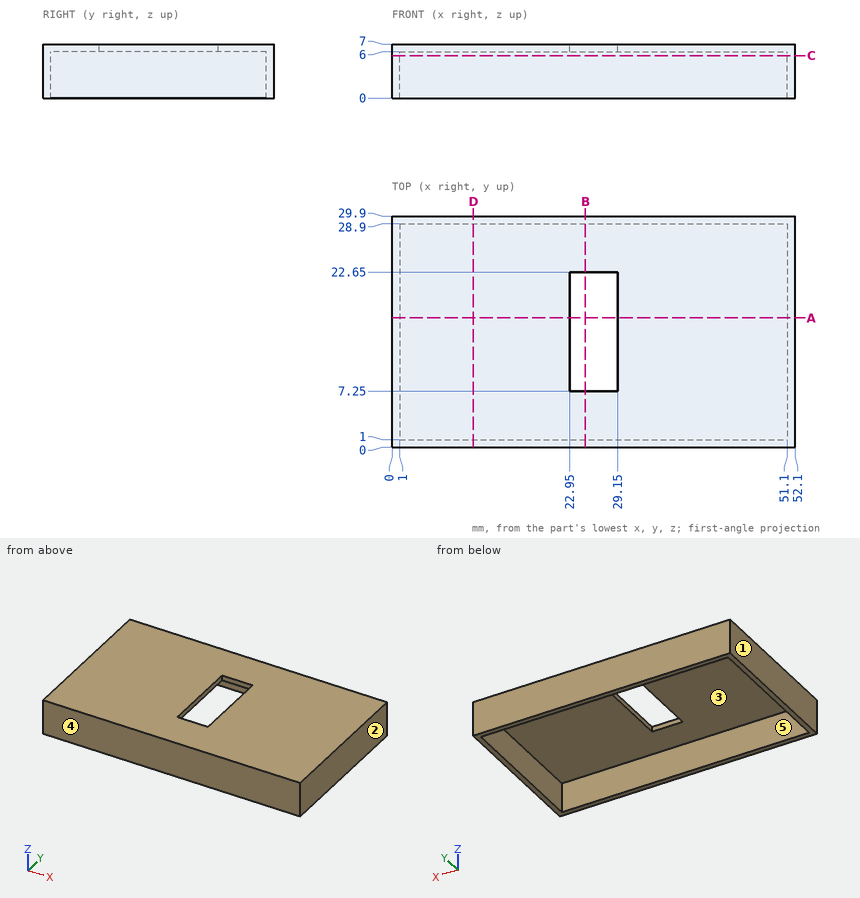
Could you check a few things on this drawing? It's one solid part, dimensions in mm from its lowest x, y, z. A direction names the side the tool comes from. Give positions to 0.01 mm unless a question says otherwise; leave off trailing zeros. Write each loop counter-clockwise with the first axis right and the second up, starting at its lowest first coordinate (ties: lowest second). Pieces come first, ordered by that corner, then holes. Notation, with made-up numbers: (-14.75, 74.25) -> (4.25, 74.25) arc R19 cw to (4.25, 93.25) -> close; hole circle Ø10 at (-18.5, 49). An arc over 180 degrees is marked (long way). Answer as a JSON object with one key per item and string values.
Q1. Will this pin go through, and if not, where does the flat tip stop? pin 1 Ø6 at (x, y) = (44, 7.5) entering from -Z.
Taken from the geometry:
{"pin 1": "stops at z = 6"}
Q2. Suppose I cut it at D-D on x = 10.5. Write out the boundary of the cut face in (y, z), then the cut area to 3 significant figures.
Taken from the geometry:
{"outline": "(0, 0) -> (1, 0) -> (1, 6) -> (28.9, 6) -> (28.9, 0) -> (29.9, 0) -> (29.9, 7) -> (0, 7) -> close", "area": "41.9 mm²"}
Q3. We'd pull the mould along X, two halves only. Please class the marked faces 1, 2 and 3: released by +X, released by -X, zero draft, split by the parting line, or undercut.
Taken from the geometry:
{"face 1": "released by -X", "face 2": "released by +X", "face 3": "undercut"}
Q4. Suppose I cut it at C-C on z = 5.5. Write out the boundary of the cut face in (x, y), then the cut area to 3 significant figures.
Taken from the geometry:
{"outline": "(0, 0) -> (52.1, 0) -> (52.1, 29.9) -> (0, 29.9) -> close; hole (1, 1) -> (51.1, 1) -> (51.1, 28.9) -> (1, 28.9) -> close", "area": "160 mm²"}
Q5. Suppose I cut it at A-A on y = 16.75. Write out the boundary of the cut face in (x, z).
Taken from the geometry:
{"outline": "(0, 0) -> (1, 0) -> (1, 6) -> (22.95, 6) -> (22.95, 7) -> (0, 7) -> close; (29.15, 6) -> (51.1, 6) -> (51.1, 0) -> (52.1, 0) -> (52.1, 7) -> (29.15, 7) -> close"}
Q6. Please list where these lines run through material, in increasing order: L1, parallel to Y at x = 48, z = 3.75; L2, parallel to X at y = 7.5, z = 5.5; L3, parallel to X at y = 14.5, z = 6.75.
Taken from the geometry:
{"L1": "y = 0 to 1, 28.9 to 29.9", "L2": "x = 0 to 1, 51.1 to 52.1", "L3": "x = 0 to 22.95, 29.15 to 52.1"}
Q7. Which directions (+Z, -Z, +X, -X, +Y, -Y) give clear straight access to the entire face, cutting with the end or side of a thin tool? Please do the marked faces 4 and 5.
Taken from the geometry:
{"face 4": "+Z, -Z, +X, -X, -Y", "face 5": "-Z"}
Q8. Suppose I cut it at B-B on x = 25. Write out the boundary of the cut face in (y, z), then the cut area to 3 significant figures.
Taken from the geometry:
{"outline": "(0, 0) -> (1, 0) -> (1, 6) -> (7.25, 6) -> (7.25, 7) -> (0, 7) -> close; (22.65, 6) -> (28.9, 6) -> (28.9, 0) -> (29.9, 0) -> (29.9, 7) -> (22.65, 7) -> close", "area": "26.5 mm²"}
